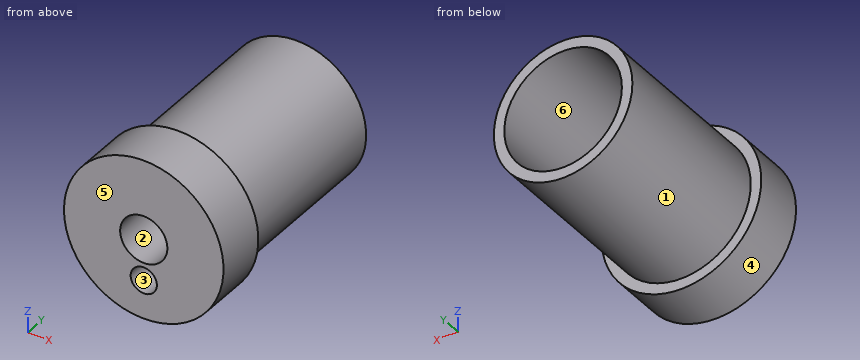
Autodesk Inventor part; units mm, degrees
ref_plane "YZ Plane" through (0, 0, 0) normal (1, 0, 0) x (0, 1, 0)
ref_plane "XZ Plane" through (0, 0, 0) normal (0, 1, 0) x (-1, 0, 0)
ref_plane "XY Plane" through (0, 0, 0) normal (0, 0, 1) x (1, 0, 0)
sketch "Sketch1" plane through (0, 0, 0) normal (0, 1, 0) x (-1, 0, 0)
  circle A0 centre (0, 0) radius 5.6
  circle A1 centre (0, 0) radius 2.25
  circle A2 centre (0, 0) radius 6.6
  circle A3 centre (0, 0) radius 7.6
  dimension "d0" = 11.2
  dimension "d1" = 4.5
  dimension "d6" = 1
  dimension "d7" = 1
extrude "Extrusion1" add sketch "Sketch1" along normal blind 5 contours A0 | A2 | A3
extrude "Extrusion3" add sketch "Sketch1" along normal blind 17 from surface at 5 contours A2
sketch "Sketch4" plane through (0, 5, 0) normal (0, 1, 0) x (1, 0, 0)
  circle A0 centre (0, 3.925) radius 1.25
  circle A1 centre (0, 0) radius 2.25
  line L0 (0, 2.25) -> (0, 5.6) construction
  circle A2 centre (0, 0) radius 5.6
  dimension "d19" = 2.5
extrude "Extrusion5" cut sketch "Sketch4" against normal up to surface (5 mm away) contours A0
properties part number "button middle part 2"
Model file for the job. Use its own axes, mm. Face numbers are marked on the shaded views. A direction names the side the tool comes from. Round coordinates to 2 decimals unless told otherwise and drop trailing zeros. Order: outer loops, then holes, each group sorted by start corner. A loop starts at its lowest first (then second) coordinate and runs counter-clockwise, first axis right, second up. Notation, with made-up numbers: M 0.5,36 L 24.5,36 A21 cw 24.5,48 Z; hole C -11.75,88 d5. An arc over 180 degrees is marked long. Use CSV: the item, a comma, the result in double quotes.
Item 1: Probe probe 1 along Z at (x, y) = (0, 3.35) (3 decimals); probe 2 along X at (y, z) = (5.5, 0.25); probe 3 along Y at (x, z) = (-3, 2.75). List the from-to ranges inside material, lowest first.
Worked answers:
probe 1,"-7.6 to -5.175, -2.675 to -2.25, 2.25 to 7.6"
probe 2,"-6.6 to -5.59, 5.59 to 6.6"
probe 3,"0 to 5"
Item 2: Saw through at B-B (z = 0). List the corners of the cut face in (x, y), plus the area to 3 significant figures.
Worked answers:
outline,"M -7.6,0 L -2.25,0 L -2.25,5 L -5.6,5 L -5.6,22 L -6.6,22 L -6.6,5 L -7.6,5 Z; M 2.25,0 L 7.6,0 L 7.6,5 L 6.6,5 L 6.6,22 L 5.6,22 L 5.6,5 L 2.25,5 Z"
area,"87.5 mm²"
Item 3: Saw through at D-D (x = -6.25). List the corners of the cut face in (y, z).
Worked answers:
outline,"M 0,-4.32 L 5,-4.32 L 5,-2.12 L 22,-2.12 L 22,2.12 L 5,2.12 L 5,4.32 L 0,4.32 Z"
Item 4: Which spindle directions (+Z, -Z, +X, -X, +Y, -Y) get a long thin tool onto all of the face, cutting with end or side? Do the marked faces 1 and 2. Say none if no direction does.
Worked answers:
face 1,"+Y"
face 2,"+Y, -Y"
Item 5: Saw through at C-C (y = 18.5). List the corners of the cut face in (x, z).
Worked answers:
outline,"C 0,0 d13.2; hole C 0,0 d11.2"
Item 6: Pin check, flat tips, straight feed: pin 1 (4 mm diameter, centred on x = 1.5, z = 0, fed in from +Y); pin 2 (9 mm diameter, centred on x = 1.5, z = -1, fed in from +Y); pin 3 (3.5 mm diameter, centred on x = 0, z = 0, fed in from +Y); pin 4 (8 mm diameter, centred on y = 15, z = 3.5, fed in from +X). Stop position of each tip, or through.
Worked answers:
pin 1,"y = 5"
pin 2,"y = 22"
pin 3,"through"
pin 4,"x = 6.6"
Item 7: Pull direction Z, two halves, no side cores. Call the marked faces 3, 4, 5 and 6: released by +Z, released by -Z, zero draft, split by the parting line, or undercut.
Worked answers:
face 3,"undercut"
face 4,"split by the parting line"
face 5,"zero draft"
face 6,"undercut"
Item 8: Saw through at A-A (x = 0). List the corners of the cut face in (y, z) (3 decimals), plus the area to 3 significant figures.
Worked answers:
outline,"M 0,-7.6 L 5,-7.6 L 5,-6.6 L 22,-6.6 L 22,-5.6 L 5,-5.6 L 5,-5.175 L 0,-5.175 Z; M 0,-2.675 L 5,-2.675 L 5,-2.25 L 0,-2.25 Z; M 0,2.25 L 5,2.25 L 5,5.6 L 22,5.6 L 22,6.6 L 5,6.6 L 5,7.6 L 0,7.6 Z"
area,"75.0 mm²"
